Answer from the drawing. Dimensions are ordinates in mm from the lowest x, y and z of the part. A direction names the side the tool comes from. Coordinates: 2 decimals unless noted, no trailing zeros. Order: outer loops, then holes, each group sorted by start corner. A loop starts at its lowest first (then second) coordinate and runs counter-clockwise, first axis right, second up. Notation, with made-up numbers: (86.5, 63) - (104.5, 63) arc R35 ccw to (104.5, 101) - close; hole circle Ø3 at (71, 86.25). An arc over 180 degrees is marked (long way). Use a Markdown table: item, result. Add a question column.
Item 1: The part is cut by section D-D, the plane x = 3.75. Give the vertices of the cut face in (y, z), then the cut area to 3 significant figures.
Item 2: The part is cut by section C-C, the plane y = 13.75. Give the vertices of the cut face in (x, z), then the cut area to 3 significant figures.
Item 3: Find the intervals of material crossed by line 1 along Z through (x, y) = (10, 13.75); line 2 along Y through (x, z) = (7, 4.5), in increasing order.
Item 4: Flat-ended cylindrical pins translate along their axes: P1, Ø1, axis at y = 7, z = 15, coming from the +X side; P2, Ø8, axis at x = 9, z = 7.5, coming from the +Y side; P3, Ø4, axis at x = 3.5, y = 3.5, coming from the -Z side. Find the tip coordinate at first contact, or state that the pin passes through.
Item 5: The part is cut by section A-A, the plane x = 10. Give the vertices of the cut face in (y, z), then the cut area to 3 significant figures.
Item 6: The part is cut by section B-B, the plane z = 11. Give the vertices of the cut face in (x, y).
Item 7: The mould has two halves that part along Z. Classify the marked faces 4, 5 and 6: released by +Z, released by -Z, zero draft, split by the parting line, or undercut.
Item 8: For the marked faces 1, 2 and 3, determine the directions among +Z, -Z, +X, -X, +Y, -Y from which every point of the face is accessible in a straight line to the end or side of a thin tool.
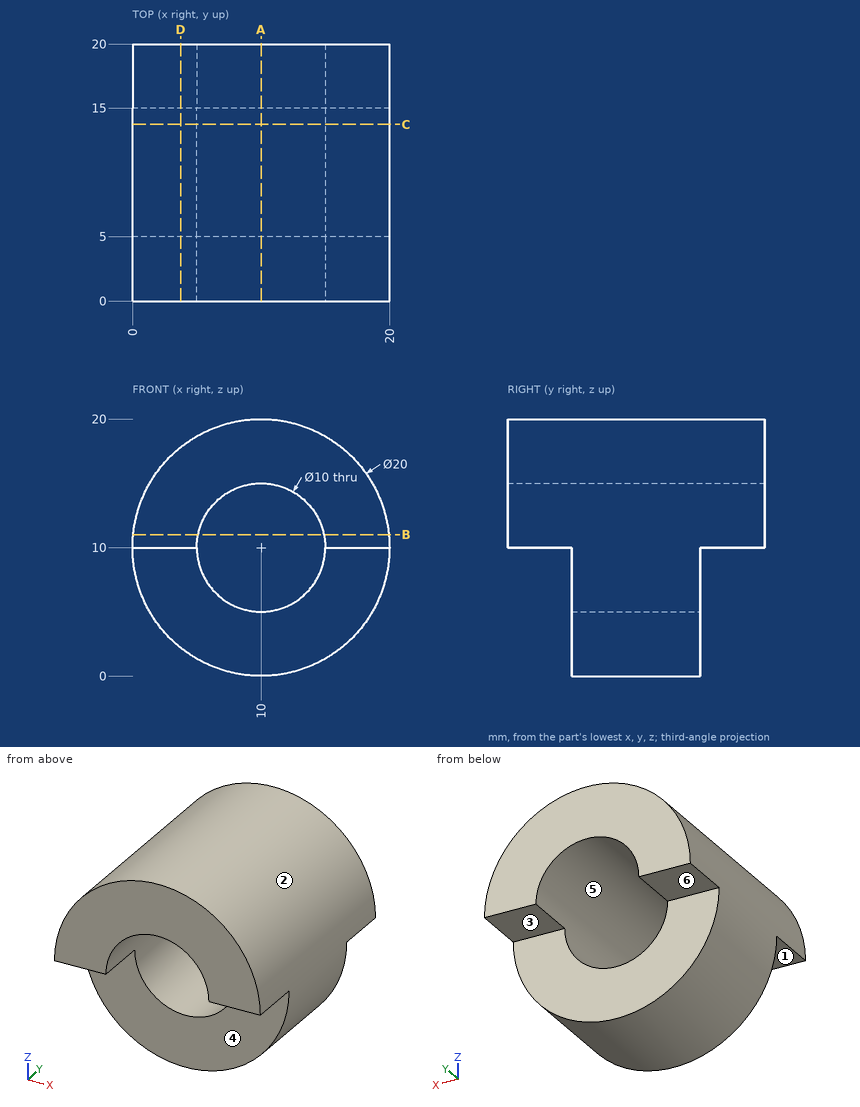
Solution:
| question | item | result |
|---|---|---|
| 1 | outline | (0, 10) - (5, 10) - (5, 2.19) - (15, 2.19) - (15, 10) - (20, 10) - (20, 17.81) - (0, 17.81) - close |
| 1 | area | 234 mm2 |
| 2 | outline | circle Ø20 at (10, 10); hole circle Ø10 at (10, 10) |
| 2 | area | 236 mm2 |
| 3 | line 1 | z = 0 to 5, 15 to 20 |
| 3 | line 2 | y = 5 to 15 |
| 4 | P1 | stops at x = 18.93 |
| 4 | P2 | stops at y = 15 |
| 4 | P3 | stops at z = 1.44 |
| 5 | outline | (0, 15) - (20, 15) - (20, 20) - (0, 20) - close; (5, 0) - (15, 0) - (15, 5) - (5, 5) - close |
| 5 | area | 150 mm2 |
| 6 | outline | (0.05, 0) - (5.1, 0) - (5.1, 20) - (0.05, 20) - close; (14.9, 0) - (19.95, 0) - (19.95, 20) - (14.9, 20) - close |
| 7 | face 4 | zero draft |
| 7 | face 5 | undercut |
| 7 | face 6 | released by -Z |
| 8 | face 1 | -Z, +X, -X, -Y |
| 8 | face 2 | +Y, -Y |
| 8 | face 3 | -Z, +X, -X, +Y |
